Job drawing, mm, ordinate dimensions from the low corner. One solid piece. Give positions to 0.01 mm unless a question says otherwise; leave off trailing zeros. Order: outer loops, then holes, each group sorted by start corner. A loop starts at its lowest first (then second) coordinate and runs counter-clockwise, first axis right, second up. Notation, with made-up numbers: (82, -13) -> (132, -13) arc R27 cw to (132, 24) -> close; hole circle Ø10 at (84.25, 64). An arc over 180 degrees is marked (long way). Use CSV: the item, a comma, the result in double quotes. Start each with the question number.
1. Cut at D-D on y = 139.5. List the corners of the cut face in (x, z), then the cut area to 3 significant figures.
2. Wall check: line 1 (Y direction, x = 130, z = 1.85); line 2 (Y direction, x = 162.5, z = 2.3); line 3 (X direction, y = 175, z = 2.35). Give the ranges that are in metal, low to high. Write a range as from..to.
3. Drop flat-ended pins along their axis: pin 1 (7.5 mm diameter, centred on x = 162.5, y = 60, fed in from -Z); pin 2 (13.5 mm diameter, centred on x = 182.5, y = 100, fed in from +Z). Give the stop position or say it passes through.
4. Cut at B-B on y = 60. List the corners of the cut face in (x, z), then the cut area to 3 significant figures.
5. Cut at C-C on y = 25. List the corners of the cut face in (x, z).
6. Cut at A-A on x = 25. List the corners of the cut face in (y, z).
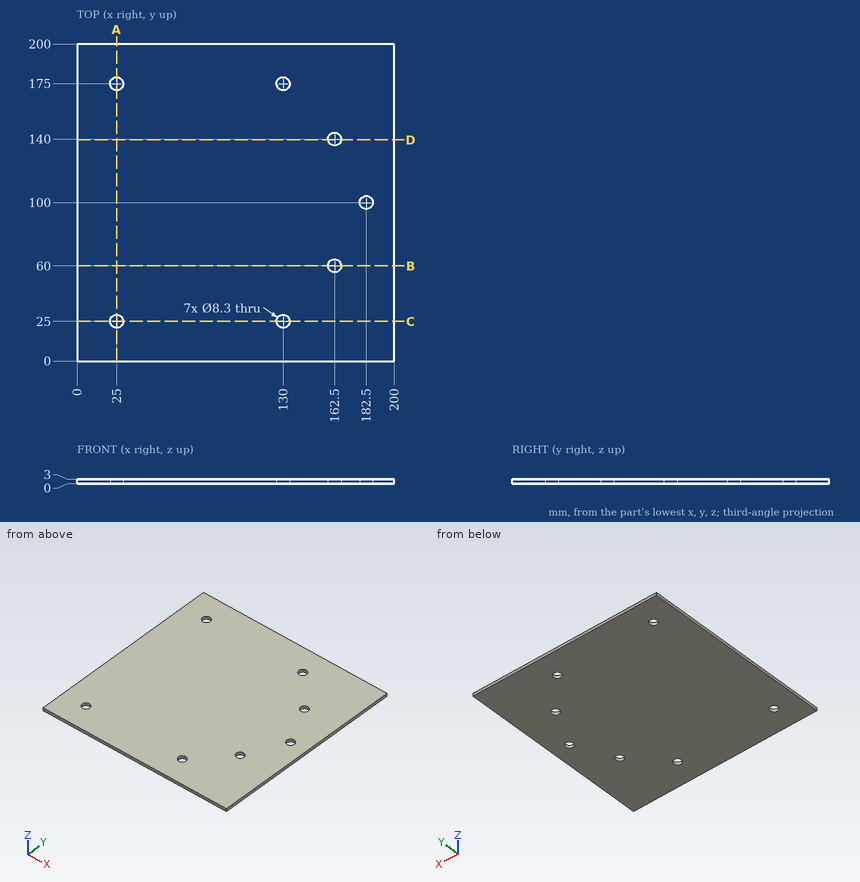
Verdict:
1,outline,"(0, 0) -> (158.38, 0) -> (158.38, 3) -> (0, 3) -> close; (166.62, 0) -> (200, 0) -> (200, 3) -> (166.62, 3) -> close"
1,area,"575 mm^2"
2,line 1,"0..20.85, 29.15..170.85, 179.15..200"
2,line 2,"0..55.85, 64.15..135.85, 144.15..200"
2,line 3,"0..20.85, 29.15..125.85, 134.15..200"
3,pin 1,"through"
3,pin 2,"z = 3"
4,outline,"(0, 0) -> (158.35, 0) -> (158.35, 3) -> (0, 3) -> close; (166.65, 0) -> (200, 0) -> (200, 3) -> (166.65, 3) -> close"
4,area,"575 mm^2"
5,outline,"(0, 0) -> (20.85, 0) -> (20.85, 3) -> (0, 3) -> close; (29.15, 0) -> (125.85, 0) -> (125.85, 3) -> (29.15, 3) -> close; (134.15, 0) -> (200, 0) -> (200, 3) -> (134.15, 3) -> close"
6,outline,"(0, 0) -> (20.85, 0) -> (20.85, 3) -> (0, 3) -> close; (29.15, 0) -> (170.85, 0) -> (170.85, 3) -> (29.15, 3) -> close; (179.15, 0) -> (200, 0) -> (200, 3) -> (179.15, 3) -> close"
